Read the model definition and answer for the solid it produces. Units are mm, in the model's axes. A direction names the side the tool comes from. Coordinates: 2 decimals unless noted, no trailing zeros. Order: outer loops, then holes, each group sorted by start corner. A loop starts at its lowest first (then second) coordinate and runs counter-clockwise, first axis right, second up. Notation, with made-up numbers: M -7,55 L 5,55 A21 cw 5,91 Z; hole C 53.5,77.5 d4. An arc over 180 degrees is marked long. Put each result on its own line as item: value.
Autodesk Inventor part; units mm, degrees
ref_plane "YZ Plane" through (0, 0, 0) normal (1, 0, 0) x (0, 1, 0)
ref_plane "XZ Plane" through (0, 0, 0) normal (0, 1, 0) x (-1, 0, 0)
ref_plane "XY Plane" through (0, 0, 0) normal (0, 0, 1) x (1, 0, 0)
sketch "Esquisse1" plane through (0, 0, 0) normal (1, 0, 0) x (0, 1, 0)
  line L0 (0, 0) -> (0, 36.6667)
  line L1 (17.5, 0) -> (17.5, 25)
  line L2 (17.5, 0) -> (11, 0)
  line L3 (17.5, 25) -> (9, 40)
  line L4 (9, 40) -> (8, 40)
  line L5 (8, 40) -> (8, 30)
  line L6 (8, 30) -> (10, 30)
  line L7 (10, 30) -> (13, 25)
  line L8 (13, 25) -> (13, 3)
  line L9 (13, 3) -> (11, 3)
  line L10 (11, 0) -> (11, 3)
  dimension "d0" = 35
  dimension "d1" = 16
  dimension "d2" = 1
  dimension "d3" = 2
  dimension "d4" = 26
  dimension "d7" = 5
  dimension "d8" = 10
  dimension "d11" = 30
  dimension "d12" = 22
  dimension "d13" = 3
revolve "Révolution1" add sketch "Esquisse1" angle 360 about axis through (0, 0, 0) along (0, 0, 1)
properties part number "blocage_recule_support_douille"
Q1. Consider line 1 along X through (y, z) = (0, 14); line 2 along X through (y, z) = (0, 2). Determine where each line is inside the solid, lowest interval first.
Answers below:
line 1: x = -17.5 to -13, 13 to 17.5
line 2: x = -17.5 to -11, 11 to 17.5
Q2. For a pull along Y with two mould halves and no side action, classify faces 4 (the face through (-9.945, -2.208, 29.687)), 5 (the face through (10.648, -13.887, 12.675)), 6 (the face through (8, -8, 0)) as +Y half, -Y half, draft (parallel to the pull), parting line (faces both ways), or undercut.
Answers below:
face 4: undercut
face 5: parting line
face 6: draft
Q3. Find section D-D on z = 32. Write down the section's boundary in (x, y).
Answers below:
outline: C 0,0 d27.07; hole C 0,0 d16
Q4. Given pin 1 (21 mm diameter, centred on x = 0, y = 0, fed in from +Z); pin 2 (5 mm diameter, centred on x = -12, z = 10, fed in from -Y); pin 3 (10 mm diameter, centred on y = 5.5, z = 11, fed in from +X); pin 4 (10 mm diameter, centred on x = -2.5, y = 0.5, fed in from -Z), each flat-ended and moving along its own axis, determine where each tip first touches the part or whether it passes through.
Answers below:
pin 1: stops at z = 40
pin 2: stops at y = -14.7
pin 3: stops at x = 17.49
pin 4: passes through
Q5. A tool of negligible diameter and unlimited length cuts with its end or side. For faces 1 (the face through (-7.81, -1.73, 34.93)), 2 (the face through (-3, -11, 3)), 3 (the face through (10.74, -2.38, 1.52)), from which of +Z, -Z, +X, -X, +Y, -Y can it reach the whole face along a straight path? Write none if from no direction.
Answers below:
face 1: +Z, -Z
face 2: none
face 3: -Z
Q6. Find section C-C on z = 13. Write down the section's boundary in (x, y), plus the area to 3 significant figures.
Answers below:
outline: C 0,0 d35; hole C 0,0 d26
area: 431 mm^2
Q7. Find section A-A on y = 0. Write down the section's boundary in (x, z), plus the area to 4 significant figures.
Answers below:
outline: M -17.5,0 L -11,0 L -11,3 L -13,3 L -13,25 L -10,30 L -8,30 L -8,40 L -9,40 L -17.5,25 Z; M 8,30 L 10,30 L 13,25 L 13,3 L 11,3 L 11,0 L 17.5,0 L 17.5,25 L 9,40 L 8,40 Z
area: 359.5 mm^2
